Autodesk Inventor part; units mm, degrees
ref_plane "YZ Plane" through (0, 0, 0) normal (1, 0, 0) x (0, 1, 0)
ref_plane "XZ Plane" through (0, 0, 0) normal (0, 1, 0) x (-1, 0, 0)
ref_plane "XY Plane" through (0, 0, 0) normal (0, 0, 1) x (1, 0, 0)
sketch "Sketch1" plane through (0, 0, 0) normal (0, 0, 1) x (1, 0, 0)
  line L0 (-50, -50) -> (50, -50)
  line L1 (50, 50) -> (-50, 50)
  line L2 (-50, 50) -> (-50, -50)
  line L3 (50, -50) -> (-50, 50) construction
  circle A0 centre (0, -43.6681) radius 2.8575
  line L4 (50, 50) -> (50, -50)
  circle A1 centre (-38.091, -38.091) radius 2.8575
  circle A2 centre (40.636, -9.3004) radius 1.5113
  circle A3 centre (45.8176, -9.3004) radius 1.5113
  circle A4 centre (40.636, 7.0318) radius 1.5113
  circle A5 centre (45.8176, 7.0318) radius 1.5113
  circle A6 centre (-45.8176, 7.0318) radius 1.5113
  circle A7 centre (-40.636, 7.0318) radius 1.5113
  circle A8 centre (-45.8176, -9.3004) radius 1.5113
  circle A9 centre (-40.636, -9.3004) radius 1.5113
  dimension "d0" = 100
  dimension "d1" = 100
  dimension "d2" = 5.715
  dimension "d8" = 5.715
  dimension "d19" = 3.0226
  dimension "d24" = 2.159
  dimension "d25" = 13.3096
extrude "Extrusion3" add sketch "Sketch1" along normal blind 25.4
properties part number "fram jp"
The listing builds one solid part. Answer for the finished solid, in the listing's coordinates (mm). Coordinates: 2 decimals unless noted, no trailing zeros. Order: outer loops, then holes, each group sorted by start corner. A loop starts at its lowest first (then second) coordinate and runs counter-clockwise, first axis right, second up. Notation, with made-up numbers: M 38,53.5 L 82,53.5 A13 cw 82,62.5 Z; hole C 0,-35 d7. An arc over 180 degrees is marked long. Use CSV: the item, a comma, the result in double quotes.
Q1. Given pin 1 Ø1.8 at (x, y) = (45.82, 7.03) entering from -Z; pin 2 Ø5 at (x, y) = (40.64, 7.03) entering from +Z, each flat-ended and moving along its own axis, determine where each tip first touches the part or whether it passes through.
Here are the results:
pin 1,"through"
pin 2,"z = 25.4"
Q2. Determine the mould class of faces 1 (the flat face through (-1, 1, 25.4)), 2 (the cylindrical face through (47.214, 7.611, 12.522)), 3 (the flat face through (-50, 1, 13)) for opening direction X: pulls with the +X half, pulls with the -X half, needs draft (parallel to the pull), parting line crosses it, or undercut.
Here are the results:
face 1,"needs draft"
face 2,"undercut"
face 3,"pulls with the -X half"
Q3. Straight lines are drawn through the part: L1, parallel to Y at x = 0, z = 17.5; L2, parallel to X at y = -9, z = 6.5; L3, parallel to X at y = -38.5, z = 19.5. For each, find the intervals that lie inside material, in ascending order.
Here are the results:
L1,"-50 to -46.53, -40.81 to 50"
L2,"-50 to -47.3, -44.34 to -42.12, -39.15 to 39.15, 42.12 to 44.34, 47.3 to 50"
L3,"-50 to -40.92, -35.26 to 50"
Q4. Section A-A (x = 0) is taken. Determine the outline of the cut face in (y, z).
Here are the results:
outline,"M -50,0 L -46.53,0 L -46.53,25.4 L -50,25.4 Z; M -40.81,0 L 50,0 L 50,25.4 L -40.81,25.4 Z"
